Here's the drawing with two shaded views (mm, measured from the low corner). I have some questions. A direction names the side the tool comes from. Give positions to 0.01 mm unless a question says otherwise; leave off trailing zeros. Write each loop counter-clockwise with the first axis right and the second up, starting at its lowest first coordinate (ties: lowest second). Pieces come first, ordered by that corner, then holes. Notation, with made-up numbers: (86.5, -34.5) -> (111.5, -34.5) arc R9 cw to (111.5, -30.5) -> close; hole circle Ø11 at (7.25, 25). An arc over 180 degrees is marked (long way). Put each result on its own line as item: value. Start each with the question number.
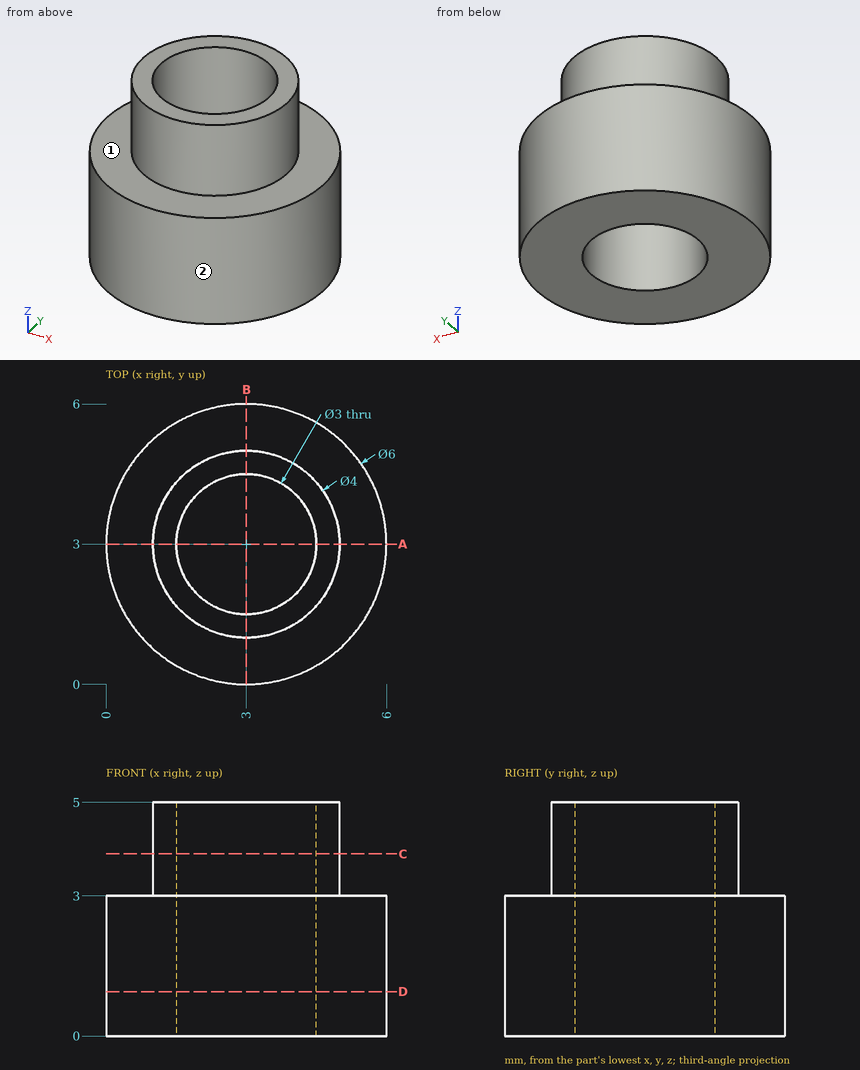
1) Which directions (+Z, -Z, +X, -X, +Y, -Y) give clear straight access to the entire face, cutting with the end or side of a thin tool? Please do the marked faces 1 and 2.
2) I need wall thicknesses on probe 1 along Y at (x, z) = (3, 1.7); probe 2 along Y at (x, z) = (3, 3.4); probe 3 along X at (y, z) = (4.05, 4.55). Which ranges of each line are inside material? Lowest first, please.
3) I want a section at A-A, the plane y = 3. Write out the boundary of the cut face in (x, z), and give its area (3 significant figures).
4) I want a section at C-C, the plane z = 3.9. Write out the boundary of the cut face in (x, y), and give its area (3 significant figures).
5) I want a section at D-D, the plane z = 0.95. Write out the boundary of the cut face in (x, y).
6) I'm going to push a flat-ended pin straight in: pin 1 Ø3 at (x, y) = (3, 2) entering from +Z. Where does the tip first touch, or does it pass through?
Established:
1. face 1: +Z
1. face 2: +Z, -Z
2. probe 1: y = 0 to 1.5, 4.5 to 6
2. probe 2: y = 1 to 1.5, 4.5 to 5
2. probe 3: x = 1.3 to 1.93, 4.07 to 4.7
3. outline: (0, 0) -> (1.5, 0) -> (1.5, 5) -> (1, 5) -> (1, 3) -> (0, 3) -> close; (4.5, 0) -> (6, 0) -> (6, 3) -> (5, 3) -> (5, 5) -> (4.5, 5) -> close
3. area: 11.0 mm2
4. outline: circle Ø4 at (3, 3); hole circle Ø3 at (3, 3)
4. area: 5.50 mm2
5. outline: circle Ø6 at (3, 3); hole circle Ø3 at (3, 3)
6. pin 1: stops at z = 5
